Part print with two shaded views. Sizes in mm from the minimum x, y, z corner. Coordinates: 2 decimals unless noted, no trailing zeros. Order: outer loops, then holes, each group sorted by start corner. A loop starts at its lowest first (then second) coordinate and runs counter-clockwise, first axis right, second up. Notation, with made-up numbers: (-31.75, 14.25) - (-20.75, 14.25) arc R12 ccw to (-20.75, 19.25) - close; hole circle Ø11 at (-20.5, -31). An arc over 180 degrees is marked (long way). Return JSON: item names as keys, results as strings.
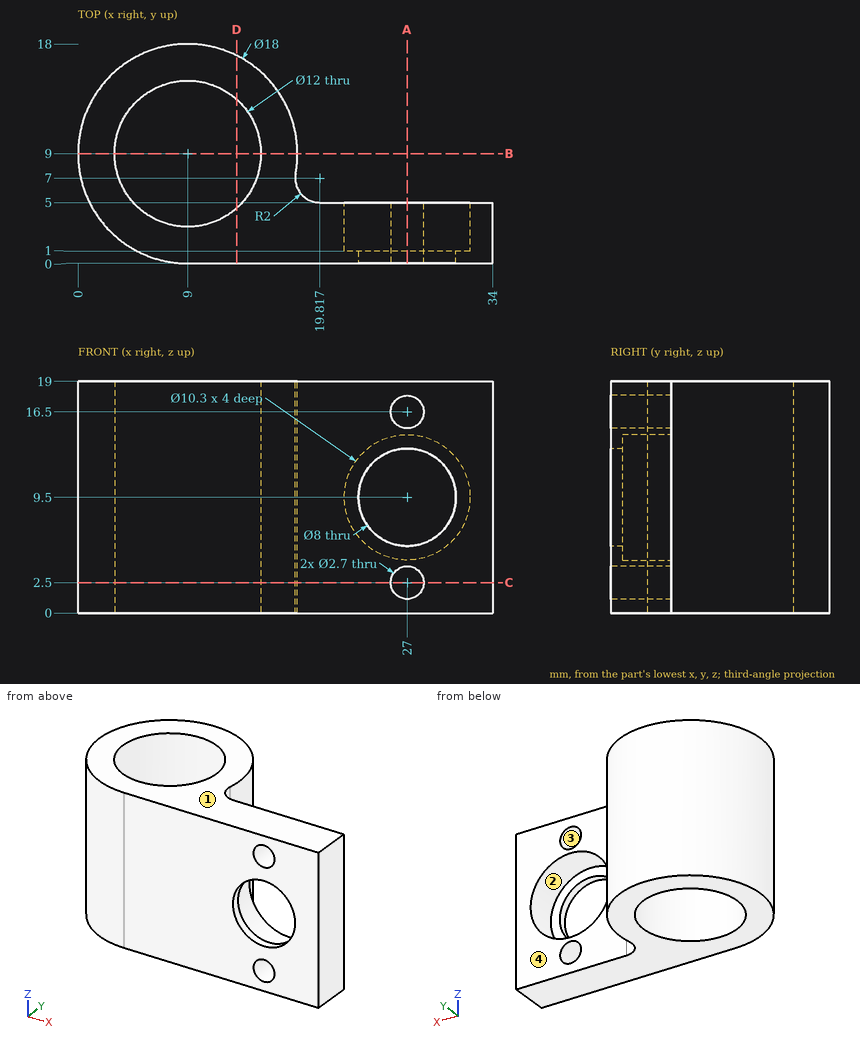
Item 1: Wall check: L1, parallel to Z at x = 27, y = 1.2; L2, parallel to X at y = 9, z = 6.25; L3, parallel to X at y = 4.25, z = 9 (1 decimal). Give the ranges that are in metal, low to high. Write a range as [from, to].
Findings below:
{"L1": "z = [0, 1.15], [3.85, 4.35], [14.65, 15.15], [17.85, 19]", "L2": "x = [0, 3], [15, 18]", "L3": "x = [1.4, 5.3], [12.7, 21.9], [32.1, 34]"}
Item 2: Band-saw the part on A-A, the plane x = 27. List the corners of the cut face in (y, z), then the cut area to 3 significant figures.
Findings below:
{"outline": "(0, 0) - (5, 0) - (5, 1.15) - (0, 1.15) - close; (0, 3.85) - (5, 3.85) - (5, 4.35) - (1, 4.35) - (1, 5.5) - (0, 5.5) - close; (0, 13.5) - (1, 13.5) - (1, 14.65) - (5, 14.65) - (5, 15.15) - (0, 15.15) - close; (0, 17.85) - (5, 17.85) - (5, 19) - (0, 19) - close", "area": "18.8 mm²"}
Item 3: Band-saw the part on C-C, the plane z = 2.5. List the corners of the cut face in (x, y).
Findings below:
{"outline": "(9, 0) - (25.65, 0) - (25.65, 5) - (19.82, 5) arc R2 cw to (17.85, 7.36) arc R9 ccw (long way) to start; (28.35, 0) - (34, 0) - (34, 5) - (28.35, 5) - close; hole circle Ø12 at (9, 9)"}
Item 4: Band-saw the part on D-D, the plane x = 13. List the corners of the cut face in (y, z).
Findings below:
{"outline": "(0, 0) - (4.53, 0) - (4.53, 19) - (0, 19) - close; (13.47, 0) - (17.06, 0) - (17.06, 19) - (13.47, 19) - close"}
Item 5: Mould opens along Z. For the marked faces 1, 2, 3 and 4 say: released by +Z, released by -Z, zero draft, split by the parting line, or undercut.
Findings below:
{"face 1": "released by +Z", "face 2": "undercut", "face 3": "undercut", "face 4": "zero draft"}
Item 6: Drop flat-ended pins along their axis: P1, Ø4.5, axis at x = 26.5, z = 5.5, coming from the +Y side; P2, Ø4, axis at x = 9.5, y = 11, coming from the +Z side; P3, Ø6, axis at y = 3, z = 9, coming from the -X side (1 decimal). Give the stop position or say it passes through.
Findings below:
{"P1": "stops at y = 5", "P2": "passes through", "P3": "stops at x = 0.5"}
Item 7: Band-saw the part on B-B, the plane y = 9. List the corners of the cut face in (x, z).
Findings below:
{"outline": "(0, 0) - (3, 0) - (3, 19) - (0, 19) - close; (15, 0) - (18, 0) - (18, 19) - (15, 19) - close"}
